For this review, use the dimensioned drawing (mm, ordinates from the lowest corner) and the shaded views. A direction names the side the tool comes from. Give positions to 0.01 mm unless a question says otherwise; leave off trailing zeros. Write each loop counter-clockwise with the first axis right and the second up, starting at its lowest first coordinate (ties: lowest second). Pieces come first, ordered by that corner, then holes. Notation, with made-up numbers: (79.25, -37.5) -> (110.25, -37.5) arc R19 cw to (110.25, -8.5) -> close; hole circle Ø1 at (-8.5, 37.25). An arc over 180 degrees is marked (long way). Return JSON: item names as keys, results as strings.
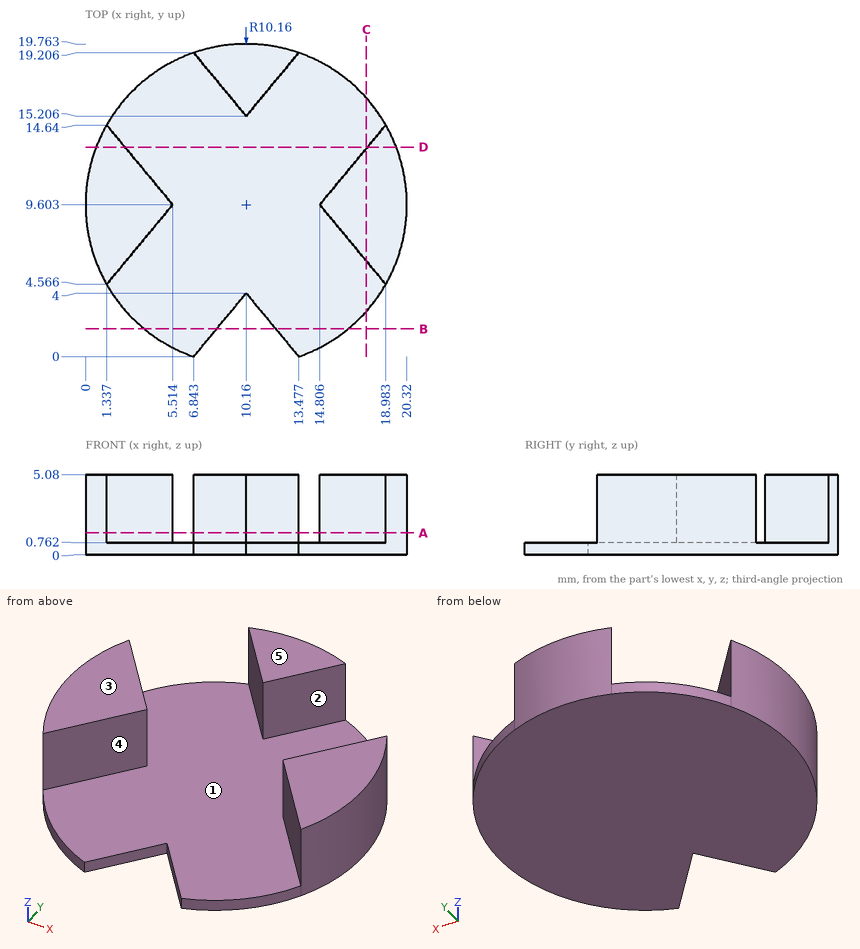
1. Add section C-C, the plane x = 17.75. State the section outline as (y, z) points.
Results found:
{"outline": "(2.85, 0) -> (16.36, 0) -> (16.36, 0.76) -> (13.15, 0.76) -> (13.15, 5.08) -> (6.05, 5.08) -> (6.05, 0.76) -> (2.85, 0.76) -> close"}
2. For pin 1 (3 mm diameter, centred on x = 7, y = 16, fed in from +Z); pin 2 (5 mm diameter, centred on x = 8.5, y = 8, fed in from -Z); pin 3 (1.5 mm diameter, centred on x = 14.5, z = 1, fed in from +Y), all flat-tipped, find the tip position at first contact; note any pin that passes through.
Results found:
{"pin 1": "stops at z = 0.76", "pin 2": "stops at z = 0", "pin 3": "stops at y = 19.09"}
3. Add section A-A, the plane z = 1.4. State the section outline as (x, y) points.
Results found:
{"outline": "(1.34, 4.57) -> (5.51, 9.6) -> (1.34, 14.64) arc R10.16 ccw to start; (6.84, 19.21) -> (10.16, 15.21) -> (13.48, 19.21) arc R10.16 ccw to start; (14.81, 9.6) -> (18.98, 4.57) arc R10.16 ccw to (18.98, 14.64) -> close"}
4. Add section B-B, the plane y = 1.75. State the section outline as (x, z) points.
Results found:
{"outline": "(3.71, 0) -> (8.29, 0) -> (8.29, 0.76) -> (3.71, 0.76) -> close; (12.03, 0) -> (16.61, 0) -> (16.61, 0.76) -> (12.03, 0.76) -> close"}
5. The part is to be moulded in two halves that separate along X. For the marked faces 1, 2 and 3, say which applies: +X half, -X half, draft (parallel to the pull), parting line (faces both ways), or undercut.
Results found:
{"face 1": "undercut", "face 2": "+X half", "face 3": "draft"}
6. For the marked faces 4 and 5, list the 3-axis set-ups (+Z, -Z, +X, -X, +Y, -Y) from which the entire face can be reached by the end or side of a thin tool; tool diameter is ignored.
Results found:
{"face 4": "+Z, -Y", "face 5": "+Z, +X, -X, +Y, -Y"}
7. To check wall thickness, follow probe 1 along Z at (x, y) = (13, 6.75); probe 2 along X at (y, z) = (9, 3.75) (1 decimal); probe 3 along X at (y, z) = (6.5, 0.8) (1 decimal). State the ranges of each line that lie inside material, in increasing order.
Results found:
{"probe 1": "z = 0 to 0.76", "probe 2": "x = 0 to 5, 15.3 to 20.3", "probe 3": "x = 0.5 to 2.9, 17.4 to 19.8"}
8. Add section D-D, the plane y = 13.25. State the section outline as (x, z) points.
Results found:
{"outline": "(0.68, 0) -> (19.64, 0) -> (19.64, 5.08) -> (17.83, 5.08) -> (17.83, 0.76) -> (2.49, 0.76) -> (2.49, 5.08) -> (0.68, 5.08) -> close"}
